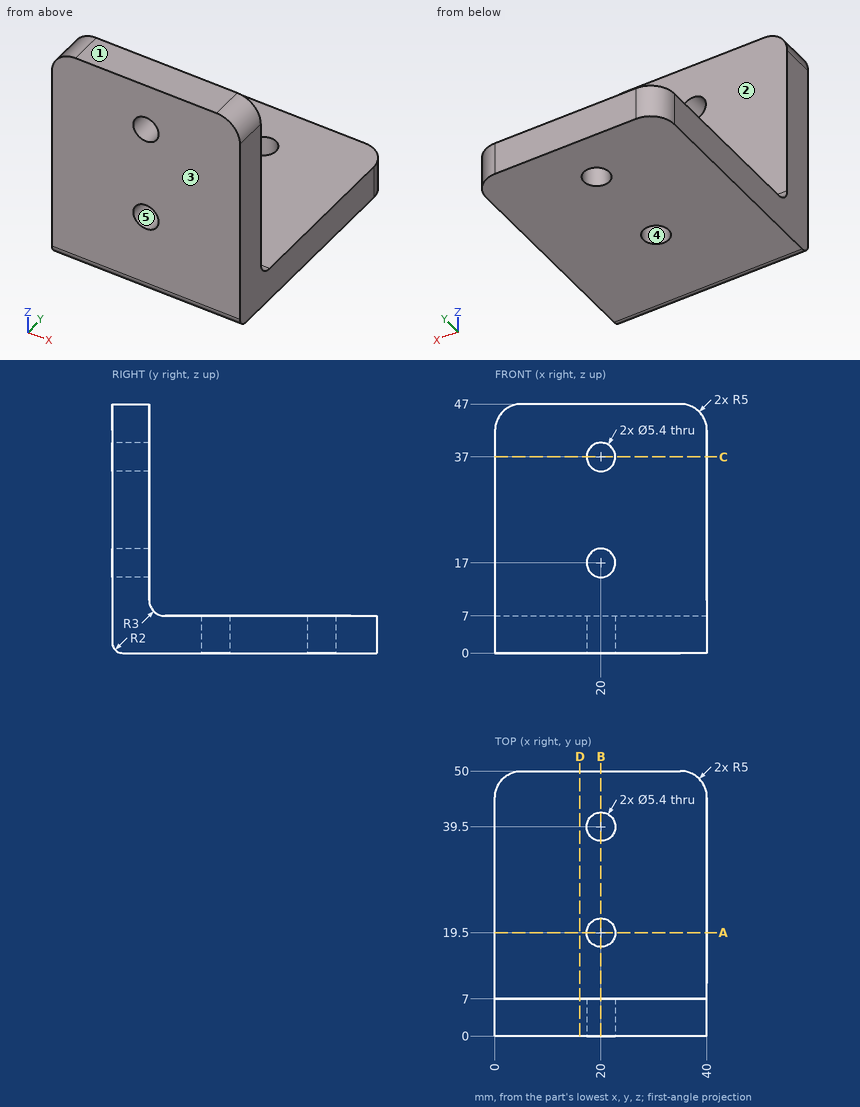
Geometry check sheet. Reference: drawing and pictorial views, mm from the part's lowest x, y, z. A direction names the side the tool comes from. Round coordinates to 2 decimals unless told otherwise and drop trailing zeros. Loops run counter-clockwise (first coordinate to the right, second up) from the corner with the lowest first, then second, coordinate; pieces in that order, holes last. Notation, with made-up numbers: M 2.5,0 L 36.5,0 A24 cw 36.5,10 Z; hole C 35.25,22.5 d10. An arc over 180 degrees is marked long. One line per item, written item: value.
(1) Thickness scan on line 1 (Z direction, x = 20, y = 4); line 2 (Y direction, x = 20, z = 4.5); line 3 (Y direction, x = 21, z = 5). Record the ranges inside material, lowest first.
Computed values:
line 1: z = 0 to 14.3, 19.7 to 34.3, 39.7 to 47
line 2: y = 0 to 16.8, 22.2 to 36.8, 42.2 to 50
line 3: y = 0 to 16.99, 22.01 to 36.99, 42.01 to 50
(2) Sectioned sample at A-A, the plane y = 19.5. Record the cut outline in (x, z), then the cut area to 3 significant figures.
Computed values:
outline: M 0,0 L 17.3,0 L 17.3,7 L 0,7 Z; M 22.7,0 L 40,0 L 40,7 L 22.7,7 Z
area: 242 mm^2
(3) Sectioned sample at B-B, the plane x = 20. Record the cut outline in (y, z).
Computed values:
outline: M 0,2 A2 ccw 2,0 L 16.8,0 L 16.8,7 L 10,7 A3 cw 7,10 L 7,14.3 L 0,14.3 Z; M 0,19.7 L 7,19.7 L 7,34.3 L 0,34.3 Z; M 0,39.7 L 7,39.7 L 7,47 L 0,47 Z; M 22.2,0 L 36.8,0 L 36.8,7 L 22.2,7 Z; M 42.2,0 L 50,0 L 50,7 L 42.2,7 Z
(4) Access from +Z, -Z, +X, -X, +Y, -Y to the whole of each face (thin tool, end or side, straight path). Record for the marked faces 1 and 2.
Computed values:
face 1: +Z, +X, -X, +Y, -Y
face 2: +Z, +X, -X, +Y
(5) Depth check by flat-ended pin: pin 1 Ø3 at (x, z) = (17.5, 12.5) entering from +Y; pin 2 Ø3 at (x, y) = (33, 32) entering from +Z; pin 3 Ø3 at (x, z) = (20, 37) entering from +Y. Enter the tip coordinate at first touch or a pass-through.
Computed values:
pin 1: stops at y = 7
pin 2: stops at z = 7
pin 3: passes through
(6) Release check for a two-part mould opening along Y. For the marked faces 3, 4 and 5 record: +Y half, -Y half, draft (parallel to the pull), parting line (faces both ways), or undercut.
Computed values:
face 3: -Y half
face 4: undercut
face 5: draft
(7) Sectioned sample at D-D, the plane x = 16. Record the cut outline in (y, z).
Computed values:
outline: M 0,2 A2 ccw 2,0 L 50,0 L 50,7 L 10,7 A3 cw 7,10 L 7,47 L 0,47 Z
